```python
from build123d import *

# Parameters (mm, degrees)
SKETCH2_W           = 0.5
SKETCH2_H           = 2.3
BOSS_EXTRUDE1_DEPTH = 6
CUT_EXTRUDE1_REACH  = 9.85
SKETCH3_W           = 2.3
SKETCH3_H           = 1.8
CUT_EXTRUDE2_START  = -0.5
SKETCH4_R           = 0.5
CUT_EXTRUDE2_DEPTH  = 0.5
CUT_EXTRUDE3_START  = -0.5
SKETCH5_R           = 0.5
CUT_EXTRUDE3_DEPTH  = 0.5
SKETCH6_W           = 10
SKETCH6_H           = 10
CUT_EXTRUDE4_DEPTH  = 8.1
BOSS_EXTRUDE2_DEPTH = 2.1


with BuildPart() as part:
    # Sketch1 → Revolve1 (revolve)
    with BuildSketch(Plane.XY):
        with BuildLine():
            Line((3.9, 0), (3.9, 8.1))
            Line((3.9, 8.1), (5.1, 8.1))
            Line((5.1, 8.1), (5.1, 11.4))
            Line((5.1, 11.4), (4.5, 11.4))
            Line((4.5, 11.4), (4.5, 12.2))
            Line((4.5, 12.2), (3.5, 12.2))
            Line((3.5, 12.2), (2.75, 11.45))
            Line((2.75, 11.45), (2.75, 3.2))
            Line((2.75, 3.2), (1.05, 3.2))
            Line((1.05, 3.2), (1.05, 8.95))
            ThreePointArc((1.05, 8.95), (0.74246212, 9.69246212), (0, 10))
            Line((0, 10), (0, 2))
            Line((0, 2), (1.3, 2))
            Line((1.3, 2), (1.3, 0))
            Line((1.3, 0), (3.9, 0))
        make_face()
    revolve(axis=Axis((0, 10, 0), (0, -1, 0)))

    # Sketch2 → Boss-Extrude1 (add)
    with BuildSketch(Plane.XZ):
        with Locations((2.5, 0)):
            Rectangle(SKETCH2_W, SKETCH2_H)
        with Locations((-2.5, 0)):
            Rectangle(SKETCH2_W, SKETCH2_H)
    extrude(amount=BOSS_EXTRUDE1_DEPTH)

    # Sketch3 → Cut-Extrude1 (cut, up to next)
    with BuildSketch(Plane.ZY.offset(2.75), mode=Mode.PRIVATE) as cut_extrude1_sk1:
        with Locations((0, -5.1)):
            Rectangle(SKETCH3_W, SKETCH3_H)
    cut_extrude1_tool1 = extrude(cut_extrude1_sk1.sketch, amount=-CUT_EXTRUDE1_REACH, mode=Mode.PRIVATE) & part.part
    add(cut_extrude1_tool1.solids().sort_by_distance((-2.75, -5.1, 0))[0], mode=Mode.SUBTRACT)

    # Sketch4 → Cut-Extrude2 (cut)
    with BuildSketch(Plane.ZY.offset(2.75).offset(CUT_EXTRUDE2_START)):
        with Locations((0, -3.2)):
            Circle(SKETCH4_R)
        with BuildLine():
            Line((-1.15, -3.2), (-1.15, -4.4))
            Line((-1.15, -4.4), (1.15, -4.4))
            Line((1.15, -4.4), (1.15, -3.2))
            ThreePointArc((1.15, -3.2), (0, -4.2), (-1.15, -3.2))
        make_face()
    extrude(amount=CUT_EXTRUDE2_DEPTH, mode=Mode.SUBTRACT)

    # Sketch5 → Cut-Extrude3 (cut)
    with BuildSketch(Plane.ZY.offset(-2.25).offset(CUT_EXTRUDE3_START)):
        with Locations((0, -5)):
            Circle(SKETCH5_R)
        with BuildLine():
            Line((-1.15, -5), (-1.15, -6.5))
            Line((-1.15, -6.5), (1.15, -6.5))
            Line((1.15, -6.5), (1.15, -5))
            ThreePointArc((1.15, -5), (0, -6), (-1.15, -5))
        make_face()
    extrude(amount=CUT_EXTRUDE3_DEPTH, mode=Mode.SUBTRACT)

    # Sketch6 → Cut-Extrude4 (cut)
    with BuildSketch(Plane.XZ):
        with Locations((0, 8.25)):
            Rectangle(SKETCH6_W, SKETCH6_H)
        with Locations((0, -8.25)):
            Rectangle(SKETCH6_W, SKETCH6_H)
    extrude(amount=-CUT_EXTRUDE4_DEPTH, mode=Mode.SUBTRACT)

    # Sketch7 → Boss-Extrude2 (add)
    with BuildSketch(Plane(origin=(0, 4.7, 0), x_dir=(-1, 0, 0), z_dir=(0, -1, 0))):
        Polygon((0, 6.350852961), (-5.5, 3.175426481), (-5.5, -3.175426481), (0, -6.350852961), (5.5, -3.175426481), (5.5, 3.175426481), align=None)
    extrude(amount=BOSS_EXTRUDE2_DEPTH)

    # Sketch9 → Cut-Revolve1 (revolve, cut)
    with BuildSketch(Plane(origin=(0, 0, 0), x_dir=(0, 0, -1), z_dir=(1, 0, 0))):
        Polygon((6.350852961, 4.1), (5.5, 4.7), (8.5, 4.7), (8.5, 2.6), (5.5, 2.6), (6.350852961, 3.2), align=None)
    revolve(axis=Axis((0, 0, 0), (0, 1, 0)), mode=Mode.SUBTRACT)


solid = part.part
```
Work out the finished part from the listing and answer in its coordinate system (mm). A direction names the side the tool comes from. Give positions to 0.01 mm unless a question says otherwise; leave off trailing zeros. Write each loop counter-clockwise with the first axis right and the second up, starting at its lowest first coordinate (ties: lowest second). Pieces come first, ordered by that corner, then holes. Notation, with made-up numbers: (79.25, -31.75) -> (112.25, -31.75) arc R23 ccw to (112.25, -19.75) -> close; hole circle Ø5 at (32.5, 47.5). An arc over 180 degrees is marked (long way). Write each question's results on one line, items separated by ' | '.
1. A tool of negligible diameter and unlimited length cuts with its end or side. For faces 1 (the cylindrical face through (1, 6.85, 0.32)), 2 (the flat face through (0, 6, 3.25)), 3 (the flat face through (-2.75, -2, 0)), from which of +Z, -Z, +X, -X, +Y, -Y can it reach the whole face along a straight path? Write none if from no direction.
Data:
face 1: +Y | face 2: +Z, +X, -X | face 3: +Z, -Z, -X, -Y
2. Determine the mould class of faces 4 (the flat face through (-1, 4.7, 1)), 5 (the cylindrical face through (-3.9, 1.3, 0.1)), 6 (the conical face through (0.01, 2.75, -5.71)) for opening direction Z: +Z half, -Z half, draft (parallel to the pull), parting line (faces both ways), or undercut.
Data:
face 4: undercut | face 5: parting line | face 6: -Z half
3. Find section B-B on y = -0.75. Determine the outline of the cut face in (x, z), and give its area (3 significant figures).
Data:
outline: (-2.75, -1.15) -> (-2.25, -1.15) -> (-2.25, 1.15) -> (-2.75, 1.15) -> close; (2.25, -1.15) -> (2.75, -1.15) -> (2.75, 1.15) -> (2.25, 1.15) -> close | area: 2.30 mm^2
4. Straight lines are drawn through the part: L1, parallel to Z at x = 0, y = 8.25; L2, parallel to Z at x = 0, y = 0.7; L3, parallel to Y at x = 2.4, z = 0. For each, find the intervals that lie inside material, in ascending order.
Data:
L1: -5.1 to -2.75, -1.05 to 1.05, 2.75 to 5.1 | L2: -3.25 to -1.3, 1.3 to 3.25 | L3: -6 to -5.5, -4.5 to 4.7
5. Find section A-A on y = 7. Determine the outline of the cut face in (x, z), and give its area (3 significant figures).
Data:
outline: (-2.16, -3.25) -> (2.16, -3.25) arc R3.9 ccw to (2.16, 3.25) -> (-2.16, 3.25) arc R3.9 ccw to start; circle Ø2.1 at (0, 0); hole circle Ø5.5 at (0, 0) | area: 23.7 mm^2
6. Each of these flat-tipped pins is pushed along its axis until it touches: pin 1 Ø0.6 at (x, y) = (2.5, -2) entering from +Z; pin 2 Ø5 at (x, y) = (-4.5, 9.5) entering from +Z; pin 3 Ø3 at (x, z) = (0, 0.5) entering from -Y. Where does it stop, or does it pass through?
Data:
pin 1: z = 1.15 | pin 2: z = 4.69 | pin 3: y = 0
